Could you check a few things on this model? Use its own coordinates, in mm. A direction names the side the tool comes from. Round coordinates to 2 decimals unless told otherwise and drop trailing zeros. Loops run counter-clockwise (first coordinate to the right, second up) from the corner with the lowest first, then second, coordinate; pieces in that order, holes last. Notation, with made-up numbers: (9, 57.25) - (42, 57.25) arc R19 cw to (42, 79.25) - close; hole circle Ø10 at (-5, 69). An arc over 180 degrees is marked (long way). Use one line per item in the form item = value.
```python
from build123d import *

# Parameters (mm, degrees)
F0_R      = 59.746411041
F1_DEPTH  = 3
F3_DEPTH  = 1
F4_W      = 55.0267398357
F4_H      = 47.7272737771
F5_DEPTH  = 0.5
F7_DEPTH  = 1
F8_R      = 2.4738185133
F9_DEPTH  = 1
F10_R     = 2.2199318272
F10_R_2   = 1.465437808
F10_R_3   = 0.9519318114
F10_R_4   = 1.4654400208
F11_DEPTH = 1


with BuildPart() as f1:
    # F0 (on Top) → F1 (new body)
    with BuildSketch(Plane.XY):
        Circle(F0_R)
    extrude(amount=F1_DEPTH)

    # F2 (on face) → F3 (join)
    with BuildSketch(Plane.XY.offset(3)):
        Polygon((32.2861000896, 29.8997331411), (-30.8823548257, 29.8997331411), (-30.8823548257, 22.0387708396), (24.14438501, 22.0387708396), (24.14438501, -25.6885029376), (-30.8823548257, -25.6885029376), (-30.8823548257, -35.7954576612), (32.2861000896, -35.7954576612), align=None)
    extrude(amount=F3_DEPTH)

    # F4 (on face) → F5 (join)
    with BuildSketch(Plane.XY.offset(3)):
        with Locations((-3.3689849079, -1.824866049)):
            Rectangle(F4_W, F4_H)
    extrude(amount=F5_DEPTH)

    # F6 (on face) → F7 (join)
    with BuildSketch(Plane.XY.offset(3.5)):
        with BuildLine():
            add(Edge.make_bspline(
                [(-7.8967735171, 4.4630197808), (-6.7472410939, 6.3631146928), (-4.2978470766, 10.3579710963), (4.9236583813, 6.7117134789), (5.0381701976, 7.1338413451), (11.9620101246, -0.915486679), (3.2320457014, -11.8590867107), (-9.7005034886, -12.6508830087), (-9.2341364863, -19.6502724984), (-8.6216118359, -22.8505288553), (-12.5728787551, -22.7759109925), (-12.7049356975, -18.6588510203), (-12.8181265408, -12.6591944575), (-26.8299925031, -9.070957377), (-26.2673376023, -3.8043012984), (-20.0692490511, -5.9986578173), (-14.7561582368, -6.4054263727), (-11.4189815971, -1.4119849747), (-9.117917068, 2.4445567946), (-7.8967735171, 4.4630197808)],
                knots=[0, 0, 0, 0, 0.0628292736, 0.1346835267, 0.143073424, 0.2136489841, 0.3010025203, 0.3856405201, 0.4441669851, 0.4844793874, 0.523851834, 0.5706012448, 0.6285825789, 0.7189345215, 0.7591710772, 0.8181193089, 0.8750291185, 0.9332567218, 1, 1, 1, 1], degree=3))
        make_face()
    extrude(amount=F7_DEPTH)

    # F8 (on face) → F9 (cut)
    with BuildSketch(Plane.XY.offset(4.5)):
        with Locations((-1.6575232148, 2.0118856337)):
            Circle(F8_R)
    extrude(amount=-F9_DEPTH, mode=Mode.SUBTRACT)

    # F10 (on face) → F11 (join)
    with BuildSketch(Plane.XY.offset(3.5)):
        with Locations((8.4812575951, 14.6018015221)):
            Circle(F10_R)
        with Locations((2.6876691263, 17.9442577064)):
            Circle(F10_R_2)
        with Locations((4.4703115709, 13.0419889465)):
            Circle(F10_R_3)
        with Locations((8.704087697, 8.8082114235)):
            Circle(F10_R_4)
    extrude(amount=F11_DEPTH)


solid = f1.part
```
1. For P1, Ø0.8, axis at y = -4, z = 3.5, coming from the -X side; P2, Ø1.5, axis at y = -19, z = 3.5, coming from the +X side; P3, Ø0.8, axis at x = -6, z = 3.5, coming from the +Y side; P4, Ø4, axis at x = -2, y = 3, coming from the +Z side, each with a flat end and sliding along its axis, tell me the tip position at first contact or that it passes through.
Solution:
P1 = -30.88
P2 = 56.83
P3 = 29.9
P4 = 4.5
2. We'd pull the mould along X, two halves only. Please class faces 1 (the face through (-2, 2, 3.5)), 2 (the face through (57, 17.9, 1.5)), 3 (the face through (-7, -6, 4.5)): +X half, -X half, draft (parallel to the pull), parting line (faces both ways), or undercut.
Solution:
face_1 = undercut
face_2 = parting line
face_3 = draft
3. If we section it at B-B, the plane x = -43: Write out the boundary of the cut face in (y, z).
Solution:
outline = (-41.48, 0) - (41.48, 0) - (41.48, 3) - (-41.48, 3) - close
4. If we section it at A-A, the plane z = 1.1: Write out the boundary of the cut face in (x, y).
Solution:
outline = circle Ø119.49 at (0, 0)
5. Please list where these lines run through material, in increasing order: line 1 along X through (y, z) = (1.5, 3.75); line 2 along Z through (x, y) = (-22, 39); line 3 along X through (y, z) = (1.5, 1.3).
Solution:
line_1 = -9.69 to -4.08, 0.76 to 8.44, 24.14 to 32.29
line_2 = 0 to 3
line_3 = -59.73 to 59.73
6. On a 3-axis mill with a long thin cutter (end or side, diameter ignored), from which of +Z, -Z, +X, -X, +Y, -Y can I reach the whole of each face in a straight line? I mean faces 4 (the face through (26, -3, 4)), 5 (the face through (-10, 4, 3.5)), 6 (the face through (3, 18, 4.5)). Say none if no direction works.
Solution:
face_4 = +Z, +X
face_5 = +Z
face_6 = +Z, +X, -X, +Y, -Y
7. If we section it at C-C, the plane x = 52.5: Write out the boundary of the cut face in (y, z).
Solution:
outline = (-28.52, 0) - (28.52, 0) - (28.52, 3) - (-28.52, 3) - close
